For this review, take the finished solid that the model builds, in its own axes (mm). Face numbers are marked on the shaded views. A direction names the side the tool comes from. Coordinates: 2 decimals unless noted, no trailing zeros. Loops run counter-clockwise (first coordinate to the right, second up) from the corner with the lowest first, then second, coordinate; pieces in that order, holes last. Notation, with made-up numbers: M 13,-15 L 66,-15 A11 ccw 66,1 Z; hole C -10.5,-11.5 d6. An arc over 180 degrees is marked long. Write item = value, one per line.
from build123d import *

# Parameters (mm, degrees)
F0_W     = 603.25
F0_H     = 347.6625
F1_DEPTH = 6.35
F2_W     = 603.25
F2_H     = 6.35
F3_DEPTH = 42.545
F4_W     = 603.25
F4_H     = 38.1
F5_DEPTH = 6.35
F6_R     = 9.525
F7_DEPTH = 55.246


with BuildPart() as f1:
    # F0 (on Top) → F1 (new body)
    with BuildSketch(Plane.XY):
        with Locations((-8.060125, 0.454914)):
            Rectangle(F0_W, F0_H)
    extrude(amount=F1_DEPTH)

    # F2 (on face) → F3 (join)
    with BuildSketch(Plane.XY.offset(6.35)):
        with Locations((-8.060125, 171.111164)):
            Rectangle(F2_W, F2_H)
    extrude(amount=F3_DEPTH)

    # F4 (on face) → F5 (join)
    with BuildSketch(Plane.XY.offset(48.895)):
        with Locations((-8.060125, 186.986164)):
            Rectangle(F4_W, F4_H)
    extrude(amount=F5_DEPTH)

    # F6 (on face) → F7 (cut, through all)
    with BuildSketch(Plane.XY.offset(55.245)):
        with Locations((-265.235125, 190.161164)):
            Circle(F6_R)
        with Locations((249.114875, 190.161164)):
            Circle(F6_R)
    extrude(amount=-F7_DEPTH, mode=Mode.SUBTRACT)


solid = f1.part
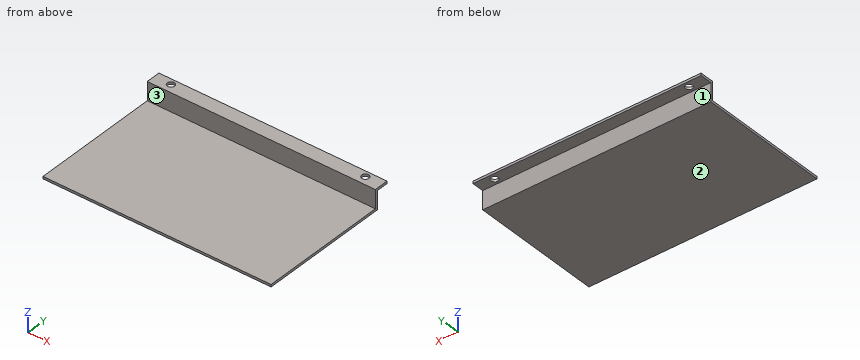
Q1. Add section B-B (z = 16.5). Write out the cut boundary in (x, y), and give its area (3 significant figures).
Solved:
outline = M -309.69,167.94 L 293.56,167.94 L 293.56,174.29 L -309.69,174.29 Z
area = 3,830 mm²
Q2. For line 1 along Z through (x, y) = (105, -131); line 2 along Y through (x, z) = (116.5, 34); line 3 along Y through (x, z) = (-90, 50), list the stretches that pass through material, from the lowest coordinate up.
Solved:
line_1 = 0 to 6.35
line_2 = 167.94 to 174.29
line_3 = 167.94 to 206.04
Q3. Add section A-A (x = -88.5). Write out the cut boundary in (y, z) (3 decimals), and give its area (3 significant figures).
Solved:
outline = M -173.376,0 L 174.286,0 L 174.286,48.895 L 206.036,48.895 L 206.036,55.245 L 167.936,55.245 L 167.936,6.35 L -173.376,6.35 Z
area = 2,720 mm²
Q4. For pin 1 Ø10 at (x, z) = (91, 9.5) entering from +Y; pin 2 Ø8 at (x, y) = (-233, 11.5) entering from +Z; pin 3 Ø15 at (x, y) = (249.11, 190.16) entering from -Z; pin 4 Ø9.5 at (x, y) = (57.5, 188.5) entering from -Z (3 decimals), all flat-tipped, find the tip position at first contact; note any pin that passes through.
Solved:
pin_1 = 174.29
pin_2 = 6.35
pin_3 = through
pin_4 = 48.895
Q5. Machinability: for the marked faces 1, 2 and 3, which of the approach directions +Z, -Z, +X, -X, +Y, -Y give a long, thin tool a straight path to every point of the face, cutting with its end or side? Answer none if there is none.
Solved:
face_1 = -Z, +X, -X, +Y
face_2 = -Z, +X, -X, +Y, -Y
face_3 = +Z, +X, -X, -Y
Q6. Add section C-C (y = -88). Write out the cut boundary in (x, z).
Solved:
outline = M -309.69,0 L 293.56,0 L 293.56,6.35 L -309.69,6.35 Z
